from build123d import *

# Parameters (mm, degrees)
SKETCH1_R          = 2.5
SKETCH1_R_2        = 1.6
SKETCH1_R_3        = 2.65
EXTRUDE1_DEPTH     = 3
CUT_EXTRUDE1_DEPTH = 3
SKETCH4_R          = 1.6
CUT_EXTRUDE2_DEPTH = 26
SKETCH5_R          = 2.75
CUT_EXTRUDE3_DEPTH = 10


with BuildPart() as part:
    # Sketch1 → Extrude1 (new body)
    with BuildSketch(Plane.XY):
        Polygon((95, -62.5), (95, 62.5), (45, 62.5), (25, 82.5), (25, 94.5), (-25, 94.5), (-25, 82.5), (-45, 62.5), (-95, 62.5), (-95, -62.5), align=None)
        with Locations((15, 85.5)):
            Circle(SKETCH1_R, mode=Mode.SUBTRACT)
        with Locations((-15, 85.5)):
            Circle(SKETCH1_R, mode=Mode.SUBTRACT)
        with Locations((-15, 55.5)):
            Circle(SKETCH1_R, mode=Mode.SUBTRACT)
        with Locations((15, 55.5)):
            Circle(SKETCH1_R, mode=Mode.SUBTRACT)
        with Locations((-75, 52.5)):
            Circle(SKETCH1_R_2, mode=Mode.SUBTRACT)
        with Locations((-55, 52.5)):
            Circle(SKETCH1_R_2, mode=Mode.SUBTRACT)
        with Locations((75, 52.5)):
            Circle(SKETCH1_R_2, mode=Mode.SUBTRACT)
        with Locations((55, 52.5)):
            Circle(SKETCH1_R_2, mode=Mode.SUBTRACT)
        with Locations((75, -52.5)):
            Circle(SKETCH1_R_2, mode=Mode.SUBTRACT)
        with Locations((55, -52.5)):
            Circle(SKETCH1_R_2, mode=Mode.SUBTRACT)
        with Locations((-55, -52.5)):
            Circle(SKETCH1_R_2, mode=Mode.SUBTRACT)
        with Locations((-75, -52.5)):
            Circle(SKETCH1_R_2, mode=Mode.SUBTRACT)
        with Locations((-26.5, -52.5)):
            Circle(SKETCH1_R_3, mode=Mode.SUBTRACT)
        with Locations((26.5, -52.5)):
            Circle(SKETCH1_R_3, mode=Mode.SUBTRACT)
        Polygon((75, -22.5), (75, 22.5), (55, 42.5), (-55, 42.5), (-75, 22.5), (-75, -22.5), (-55, -42.5), (55, -42.5), align=None, mode=Mode.SUBTRACT)
    extrude(amount=EXTRUDE1_DEPTH)

    # Sketch2 → Cut-Extrude1 (cut)
    with BuildSketch(Plane.XY.offset(3)):
        with BuildLine():
            ThreePointArc((90, -37.6), (91.6, -36), (90, -34.4))
            ThreePointArc((90, -34.4), (88.4, -36), (90, -37.6))
        make_face()
        with BuildLine():
            ThreePointArc((80, -37.6), (81.6, -36), (80, -34.4))
            ThreePointArc((80, -34.4), (78.4, -36), (80, -37.6))
        make_face()
        with BuildLine():
            ThreePointArc((90, 34.4), (91.6, 36), (90, 37.6))
            ThreePointArc((90, 37.6), (88.4, 36), (90, 34.4))
        make_face()
        with BuildLine():
            ThreePointArc((80, 34.4), (81.6, 36), (80, 37.6))
            ThreePointArc((80, 37.6), (78.4, 36), (80, 34.4))
        make_face()
    extrude(amount=-CUT_EXTRUDE1_DEPTH, mode=Mode.SUBTRACT)

    # Sketch4 → Cut-Extrude2 (cut)
    with BuildSketch(Plane.XY.offset(3)):
        with Locations((-80, -36)):
            Circle(SKETCH4_R)
        with Locations((-90, -36)):
            Circle(SKETCH4_R)
        with Locations((-80, 36)):
            Circle(SKETCH4_R)
        with Locations((-90, 36)):
            Circle(SKETCH4_R)
    extrude(amount=-CUT_EXTRUDE2_DEPTH, mode=Mode.SUBTRACT)

    # Sketch5 → Cut-Extrude3 (cut)
    with BuildSketch(Plane.XY.offset(3)):
        with Locations((-87.5, -55)):
            Circle(SKETCH5_R)
        with Locations((-87.5, -30)):
            Circle(SKETCH5_R)
        with Locations((-87.5, 30)):
            Circle(SKETCH5_R)
        with Locations((-87.5, 55)):
            Circle(SKETCH5_R)
    extrude(amount=-CUT_EXTRUDE3_DEPTH, mode=Mode.SUBTRACT)


solid = part.part
The model under review builds one solid part; all positions refer to its coordinate system, in mm. A direction names the side the tool comes from. Give positions to 0.01 mm unless a question says otherwise; leave off trailing zeros. Order: outer loops, then holes, each group sorted by start corner. A loop starts at its lowest first (then second) coordinate and runs counter-clockwise, first axis right, second up. Notation, with made-up numbers: M 54,14.5 L 60,14.5 A18 cw 60,49.5 Z; hole C 24.5,88 d3. An arc over 180 degrees is marked long. Answer in a Markdown table with one row per item. Add a question column.
1. Add section B-B on x = -65. State the section outline as (y, z) points.
2. Add section D-D on y = 30. State the section outline as (x, z) points, plus the area to 4 significant figures.
3. For pin 1 Ø1.5 at (y, z) = (88.5, 2) entering from -X; pin 2 Ø4 at (x, y) = (26.5, -52.5) entering from -Z; pin 3 Ø0.9 at (y, z) = (87, 1) entering from +X, all flat-tipped, find the tip position at first contact; note any pin that passes through.
4. Add section C-C on x = 15. State the section outline as (y, z) points, plus the area to 3 significant figures.
5. Add section A-A on y = 0. State the section outline as (x, z) points, plus the area to 3 significant figures.
6. Mouldability with a two-part tool opening along X and no side actions: class faces 3 (the flat face through (-34.9, 72.6, 1.5)), 4 (the cylindrical face through (26.16, -49.87, 1.48)), 5 (the flat face through (65.1, 32.4, 1.5)), 6 (the flat face through (-1, 52, 3)) as released by +X, released by -X, zero draft, split by the parting line, or undercut.
7. Machinability: for faces 1 (the flat face through (64.9, -32.6, 1.5)), 2 (the flat face through (-1, 52, 0)), which of the approach directions +Z, -Z, +X, -X, +Y, -Y give a long, thin tool a straight path to every point of the face, cutting with its end or side? Answer none if there is none.
8. To check wall thickness, follow line 1 along Y through (x, z) = (55, 1.25); line 2 along Y through (x, z) = (80, 2.45); line 3 along Y through (x, z) = (-87.5, 2.2). State the ranges of each line that lie inside material, in increasing order.
The answers:
| question | item | result |
|---|---|---|
| 1 | outline | M -62.5,0 L -32.5,0 L -32.5,3 L -62.5,3 Z; M 32.5,0 L 62.5,0 L 62.5,3 L 32.5,3 Z |
| 2 | outline | M -95,0 L -90.25,0 L -90.25,3 L -95,3 Z; M -84.75,0 L -67.5,0 L -67.5,3 L -84.75,3 Z; M 67.5,0 L 95,0 L 95,3 L 67.5,3 Z |
| 2 | area | 148.5 mm2 |
| 3 | pin 1 | x = -25 |
| 3 | pin 2 | through |
| 3 | pin 3 | x = 25 |
| 4 | outline | M -62.5,0 L -42.5,0 L -42.5,3 L -62.5,3 Z; M 42.5,0 L 53,0 L 53,3 L 42.5,3 Z; M 58,0 L 83,0 L 83,3 L 58,3 Z; M 88,0 L 94.5,0 L 94.5,3 L 88,3 Z |
| 4 | area | 186 mm2 |
| 5 | outline | M -95,0 L -75,0 L -75,3 L -95,3 Z; M 75,0 L 95,0 L 95,3 L 75,3 Z |
| 5 | area | 120 mm2 |
| 6 | face 3 | released by -X |
| 6 | face 4 | undercut |
| 6 | face 5 | undercut |
| 6 | face 6 | zero draft |
| 7 | face 1 | +Z, -Z |
| 7 | face 2 | -Z, +X, -X, +Y, -Y |
| 8 | line 1 | -62.5 to -54.1, -50.9 to -42.5, 42.5 to 50.9, 54.1 to 62.5 |
| 8 | line 2 | -62.5 to -37.6, -34.4 to 34.4, 37.6 to 62.5 |
| 8 | line 3 | -62.5 to -57.75, -52.25 to -32.75, -27.25 to 27.25, 32.75 to 52.25, 57.75 to 62.5 |
